from build123d import *

# Parameters (mm, degrees)
SALIENTE_EXTRUIR1_DEPTH = 126
CROQUIS2_R              = 3
CORTAR_EXTRUIR3_DEPTH   = 63


with BuildPart() as part:
    # Croquis1 → Saliente-Extruir1 (new body)
    with BuildSketch(Plane.XY):
        Polygon((0, 0), (3, 0), (3, -15), (-22, -15), (-22, -12), (0, -12), align=None)
    extrude(amount=SALIENTE_EXTRUIR1_DEPTH)

    # Croquis2 → Cortar-Extruir3 (cut, symmetric)
    with BuildSketch(Plane(origin=(3, 0, 0), x_dir=(0, 0, -1), z_dir=(1, 0, 0))):
        with Locations((-113.5, -7.5)):
            Circle(CROQUIS2_R)
        with Locations((-101, -7.5)):
            Circle(CROQUIS2_R)
        with Locations((-88.5, -7.5)):
            Circle(CROQUIS2_R)
        with Locations((-12.5, -7.5)):
            Circle(CROQUIS2_R)
        with Locations((-25, -7.5)):
            Circle(CROQUIS2_R)
        with Locations((-37.5, -7.5)):
            Circle(CROQUIS2_R)
    extrude(amount=CORTAR_EXTRUIR3_DEPTH, both=True, mode=Mode.SUBTRACT)


solid = part.part
Here's how the part is built. I have some questions about the finished solid (model axes, mm). A direction names the side the tool comes from. Give positions to 0.01 mm unless a question says otherwise; leave off trailing zeros. Order: outer loops, then holes, each group sorted by start corner. A loop starts at its lowest first (then second) coordinate and runs counter-clockwise, first axis right, second up. Notation, with made-up numbers: (42.5, 26) -> (64.5, 26) arc R24 ccw to (64.5, 48) -> close; hole circle Ø3 at (28.25, 51.25). An arc over 180 degrees is marked (long way). One line per item, written item: value. Start each with the question number.
1. Imagine slicing it at A-A, the plane y = -7.5. List the corners of the cut face in (x, z) for me, plus the area to 3 significant figures.
2. For faces 4 (the face through (0, -6, 62)), 5 (the face through (1.52, -6.6, 110.64)), which set-ups out of +Z, -Z, +X, -X, +Y, -Y let a thin tool reach every point of the face, with its end or its side?
3. Imagine slicing it at C-C, the plane z = 59.5. List the corners of the cut face in (x, y) for me, plus the area to 3 significant figures.
4. Imagine slicing it at D-D, the plane z = 12. List the corners of the cut face in (x, y) for me, plus the area to 3 significant figures.
5. Imagine slicing it at B-B, the plane z = 25. List the corners of the cut face in (x, y) for me.
6. I need wall thicknesses on probe 1 along Y at (x, z) = (1.5, 101); probe 2 along X at (y, z) = (-8.5, 80); probe 3 along Y at (x, z) = (-15.5, 22). Which ranges of each line are inside material? Lowest first, please. Write a range as from..to.
7. We'd pull the mould along Y, two halves only. Please class faces 1 (the face through (-11, -12, 62)), 2 (the face through (1.5, -7.4, 40.5)), 3 (the face through (-4.8, -12.5, 126)): released by +Y, released by -Y, zero draft, split by the parting line, or undercut.
8. Will these pins go through, and if not, where does the flat tip stop? pin 1 Ø8 at (y, z) = (-7, 51.5) entering from -X; pin 2 Ø1 at (x, z) = (-16, 56.5) entering from +Y; pin 3 Ø5 at (y, z) = (-7.5, 88.5) entering from +X.
Values follow:
1. outline: (0, 0) -> (3, 0) -> (3, 9.5) -> (0, 9.5) -> close; (0, 15.5) -> (3, 15.5) -> (3, 22) -> (0, 22) -> close; (0, 28) -> (3, 28) -> (3, 34.5) -> (0, 34.5) -> close; (0, 40.5) -> (3, 40.5) -> (3, 85.5) -> (0, 85.5) -> close; (0, 91.5) -> (3, 91.5) -> (3, 98) -> (0, 98) -> close; (0, 104) -> (3, 104) -> (3, 110.5) -> (0, 110.5) -> close; (0, 116.5) -> (3, 116.5) -> (3, 126) -> (0, 126) -> close
1. area: 270 mm2
2. face 4: +Z, -Z, -X, +Y
2. face 5: +X, -X
3. outline: (-22, -15) -> (3, -15) -> (3, 0) -> (0, 0) -> (0, -12) -> (-22, -12) -> close
3. area: 111 mm2
4. outline: (-22, -15) -> (3, -15) -> (3, -10.46) -> (0, -10.46) -> (0, -12) -> (-22, -12) -> close; (0, -4.54) -> (3, -4.54) -> (3, 0) -> (0, 0) -> close
4. area: 93.3 mm2
5. outline: (-22, -15) -> (3, -15) -> (3, -10.5) -> (0, -10.5) -> (0, -12) -> (-22, -12) -> close; (0, -4.5) -> (3, -4.5) -> (3, 0) -> (0, 0) -> close
6. probe 1: y = -15..-10.5, -4.5..0
6. probe 2: x = 0..3
6. probe 3: y = -15..-12
7. face 1: released by +Y
7. face 2: undercut
7. face 3: zero draft
8. pin 1: stops at x = 0
8. pin 2: stops at y = -12
8. pin 3: passes through
